```python
from build123d import *

# Parameters (mm, degrees)
F1_DEPTH = 2.5
F3_DEPTH = 2


with BuildPart() as f1:
    # F0 (on Front) → F1 (new body)
    with BuildSketch(Plane.XZ):
        with BuildLine():
            Line((6.5, -13), (6.5, 0))
            ThreePointArc((6.5, 0), (0, 6.5), (-6.5, 0))
            Line((-6.5, 0), (-6.5, -17))
            Line((-6.5, -17), (2.5, -17))
            Line((2.5, -17), (6.5, -13))
        make_face()
        with BuildLine():
            Line((-5.5, -16), (-5.5, 0))
            ThreePointArc((-5.5, 0), (0, 5.5), (5.5, 0))
            Line((5.5, 0), (5.5, -12.585786))
            Line((5.5, -12.585786), (2.085786, -16))
            Line((2.085786, -16), (-5.5, -16))
        make_face(mode=Mode.SUBTRACT)
    extrude(amount=F1_DEPTH)

    # F2 (on face) → F3 (cut)
    with BuildSketch(Plane.XZ.offset(2.5)):
        Polygon((6.5, -12.585786), (5.5, -12.585786), (2.085786, -16), (2.085786, -17), (2.5, -17), (6.5, -13), align=None)
    extrude(amount=-F3_DEPTH, mode=Mode.SUBTRACT)


solid = f1.part
```
Geometry: final body of the model. Coordinates: model frame, mm. A direction names the side the tool comes from. Coordinates: 2 decimals unless noted, no trailing zeros. Order: outer loops, then holes, each group sorted by start corner. A loop starts at its lowest first (then second) coordinate and runs counter-clockwise, first axis right, second up. Notation, with made-up numbers: (-3.5, 76.5) -> (22.5, 76.5) arc R18 cw to (22.5, 98.5) -> close; hole circle Ø9 at (-32, 47.5). An arc over 180 degrees is marked (long way). Use CSV: the item, a comma, the result in double quotes.
1) Line query: line 1 (Z direction, x = 0.25, y = -1.2); line 2 (X direction, y = -0.7, z = -10.75); line 3 (Z direction, x = -6, y = -2.3). Output: solid intervals per line, ascending.
Findings:
line 1,"z = -17 to -16, 5.49 to 6.5"
line 2,"x = -6.5 to -5.5, 5.5 to 6.5"
line 3,"z = -17 to 2.5"
2) Section C-C on y = -0.85. Output: boundary loops of the cut face in (x, z).
Findings:
outline,"(-6.5, -17) -> (2.09, -17) -> (2.09, -16) -> (-5.5, -16) -> (-5.5, 0) arc R5.5 cw to (5.5, 0) -> (5.5, -12.59) -> (6.5, -12.59) -> (6.5, 0) arc R6.5 ccw to (-6.5, 0) -> close"
3) Pin query (flat end, axial travel): pin 1 Ø1.2 at (x, y) = (-1.5, -1) entering from +Z; pin 2 Ø1.3 at (x, z) = (4.5, -15) entering from -Y; pin 3 Ø0.8 at (x, y) = (6, -1) entering from -Z. Return the tip coordinate at first contact, or that it passes through.
Findings:
pin 1,"stops at z = 6.44"
pin 2,"stops at y = -0.5"
pin 3,"stops at z = -12.59"
4) Section A-A on z = -12. Output: boundary loops of the cut face in (x, y), then the cut area to 3 significant figures.
Findings:
outline,"(-6.5, -2.5) -> (-5.5, -2.5) -> (-5.5, 0) -> (-6.5, 0) -> close; (5.5, -2.5) -> (6.5, -2.5) -> (6.5, 0) -> (5.5, 0) -> close"
area,"5.00 mm^2"
5) Section B-B on x = 0. Output: boundary loops of the cut face in (y, z), then the cut area to 3 significant figures.
Findings:
outline,"(-2.5, -17) -> (0, -17) -> (0, -16) -> (-2.5, -16) -> close; (-2.5, 5.5) -> (0, 5.5) -> (0, 6.5) -> (-2.5, 6.5) -> close"
area,"5.00 mm^2"
6) Mould query, pull axis Z, two halves, no side actions, for faces 1 (the cylindrical face through (-0.1, -1.2, 5.5)), 2 (the flat face through (6.5, -1, -7)), 3 (the flat face through (6, -2, -12.586)). Classes: +Z half, -Z half, draft (parallel to the pull), parting line (faces both ways), or undercut.
Findings:
face 1,"undercut"
face 2,"draft"
face 3,"-Z half"
7) Access query for faces 4 (the flat face through (5.5, -1, -6)), 5 (the flat face through (4.5, -0.2, -15)), 6 (the flat face through (2.086, -1.5, -16.5)). Directions: +Z, -Z, +X, -X, +Y, -Y. A direction counts if a zero-diameter tool reaches every point of the face in a straight line with its end or side. Return the directions, or none.
Findings:
face 4,"+Y, -Y"
face 5,"-Z, +X, +Y, -Y"
face 6,"-Z, +X, -Y"
